Autodesk Inventor part; units mm, degrees
ref_plane "YZ Plane" through (0, 0, 0) normal (1, 0, 0) x (0, 1, 0)
ref_plane "XZ Plane" through (0, 0, 0) normal (0, 1, 0) x (-1, 0, 0)
ref_plane "XY Plane" through (0, 0, 0) normal (0, 0, 1) x (1, 0, 0)
sketch "Sketch1" plane through (0, 0, 0) normal (0, 0, 1) x (1, 0, 0)
  line L0 (0, 0) -> (60, 0)
  line L1 (60, 0) -> (60, 60)
  line L2 (60, 60) -> (0, 60)
  line L3 (0, 60) -> (0, 0)
  dimension "d0" = 60
  dimension "d1" = 60
extrude "Extrusion1" add sketch "Sketch1" along normal blind 22
sketch "Sketch2" plane through (0, 0, 0) normal (0, 0, -1) x (-1, 0, 0)
  line L0 (0, 10.6066) -> (-10.6066, 0)
  line L1 (0, 10.6066) -> (0, 0)
  line L2 (0, 0) -> (-10.6066, 0)
  line L3 (0, 60) -> (-10.6066, 60)
  line L4 (-10.6066, 60) -> (0, 49.3934)
  line L5 (0, 49.3934) -> (0, 60)
  line L6 (-49.3934, 60) -> (-60, 60)
  line L7 (-60, 60) -> (-60, 49.3934)
  line L8 (-49.3934, 60) -> (-60, 49.3934)
  line L9 (-49.3934, 0) -> (-60, 0)
  line L10 (-60, 0) -> (-60, 10.6066)
  line L11 (-49.3934, 0) -> (-60, 10.6066)
  dimension "d4" = 15
  dimension "d7" = 15
  dimension "d8" = 15
  dimension "d9" = 15
extrude "Extrusion2" cut sketch "Sketch2" against normal blind 13
sketch "Sketch7" plane through (0, 0, 22) normal (0, 0, 1) x (1, 0, 0)
  circle A0 centre (45.5887, 39) radius 8 construction
  circle A1 centre (14.4113, 39) radius 8 construction
  line L0 (22, 49.3156) -> (26.1411, 33.8608) construction
  line L1 (26.1411, 33.8608) -> (16.4818, 31.2726)
  line L2 (12.3407, 46.7274) -> (22, 49.3156)
  line L3 (33.8589, 33.8608) -> (38, 49.3156) construction
  line L4 (38, 49.3156) -> (47.6593, 46.7274)
  line L5 (33.8589, 33.8608) -> (43.5182, 31.2726)
  line L6 (22, 49.3156) -> (38, 49.3156) construction
  line L7 (26.1411, 33.8608) -> (33.8589, 33.8608)
  arc A2 (12.3407, 46.7274) -> (16.4818, 31.2726) centre (14.4113, 39) ccw
  arc A3 (43.5182, 31.2726) -> (47.6593, 46.7274) centre (45.5887, 39) ccw
  line L8 (60, 60) -> (0, 60)
  arc A4 (38, 49.3156) -> (22, 49.3156) centre (30, 19.4592) ccw
  point P0 (0, 0)
  point P1 (30, 49.3156)
  point P2 (30, 60)
  dimension "d28" = 16
  dimension "d29" = 16
  dimension "d30" = 16
  dimension "d31" = 10
  dimension "d32" = 10
  dimension "d33" = 16
  dimension "d34" = 16
  dimension "d36" = 75
  dimension "d37" = 21
extrude "Extrusion7" add sketch "Sketch7" along normal blind 34
sketch "Sketch8" plane through (10.6066, 0, 13) normal (-0.7071, -0.7071, 0) x (-0.7071, 0.7071, 0)
  circle A0 centre (7.5, 9) radius 1.5
  line L0 (0, 13) -> (15, 13)
  point P0 (7.5, 13)
  point P1 (7.5, 13)
  dimension "d40" = 3
  dimension "d41" = 4
extrude "Extrusion8" cut sketch "Sketch8" against normal through all
sketch "Sketch9" plane through (60, 10.6066, 13) normal (0.7071, -0.7071, 0) x (-0.7071, -0.7071, 0)
  circle A0 centre (7.5, 9) radius 1.5
  line L0 (0, 13) -> (15, 13)
  point P0 (49.9264, 13)
  point P1 (7.5, 13)
  dimension "d44" = 3
  dimension "d45" = 4
extrude "Extrusion9" cut sketch "Sketch9" against normal through all
sketch "Sketch10" plane through (0, 0, 56) normal (0, 0, 1) x (1, 0, 0)
  line L0 (22, 49.3156) -> (12.3407, 46.7274) construction
  arc A0 (12.3407, 46.7274) -> (16.4818, 31.2726) centre (14.4113, 39) ccw construction
  line L1 (16.4818, 31.2726) -> (26.1411, 33.8608) construction
  line L2 (26.1411, 33.8608) -> (33.8589, 33.8608) construction
  line L3 (33.8589, 33.8608) -> (43.5182, 31.2726) construction
  arc A1 (43.5182, 31.2726) -> (47.6593, 46.7274) centre (45.5887, 39) ccw construction
  line L4 (47.6593, 46.7274) -> (38, 49.3156) construction
  arc A2 (38, 49.3156) -> (22, 49.3156) centre (30, 19.4592) ccw construction
  circle A3 centre (14.4113, 39) radius 1.75
  circle A4 centre (45.5887, 39) radius 1.75
  circle A5 centre (30, 46.8608) radius 1.75
  point P0 (0, 0)
  point P1 (30, 33.8608)
  dimension "d48" = 3.5
  dimension "d49" = 3.5
  dimension "d50" = 3.5
  dimension "d51" = 13
extrude "Extrusion10" cut sketch "Sketch10" against normal blind 29
properties part number "Base" material "ABS Plastic"
CAD build for the part. Positions are in the model's coordinates, mm. A direction names the side the tool comes from. Give positions to 0.01 mm unless a question says otherwise; leave off trailing zeros. Write each loop counter-clockwise with the first axis right and the second up, starting at its lowest first coordinate (ties: lowest second). Pieces come first, ordered by that corner, then holes. Notation, with made-up numbers: M -25,27.5 L 19,27.5 A31 cw 19,60.5 Z; hole C 2.25,82.25 d11. An arc over 180 degrees is marked long. Return JSON: item names as keys, results as strings. Group by question number.
(1) Mould opens along X. For faces 1 (the face through (3, 3, 13)), 2 (the face through (17.254, 41.605, 2.735)), 3 (the face through (42.76, 48.04, 38.76)), 4 (the face through (14, 37.3, 41.7)) say: pulls with the +X half, pulls with the -X half, needs draft (parallel to the pull), parting line crosses it, or undercut.
(2) Band-saw the part on A-A (z = 33.5). Give the cut face in (x, y).
(3) Band-saw the part on B-B (y = 39). State how many separate pieces and enclosed holes the cut face has, and give its area (3 significant figures).
(4) 3-axis set-ups, long thin cutter, end or side, ignore diameter. For faces 5 (the face through (46, 39, 27)), 6 (the face through (57, 3, 13)), 7 (the face through (29.89, 50.37, 38.76)), 8 (the face through (56, 56, 13)): which of +Z, -Z, +X, -X, +Y, -Y reach the whole face in a straight line?
(5) Flat gauge pins, fed straight in: pin 1 Ø4 at (x, z) = (39.5, 43) entering from +Y; pin 2 Ø1.5 at (x, z) = (41, 34.5) entering from +Y; pin 3 Ø1.5 at (x, z) = (34.5, 42.5) entering from -Y. Where does each tip first touch, or does it go through?
(6) Drill centre lines: L1, parallel to Y at x = 30, z = 50; L2, parallel to Z at x = 54, y = 6; L3, parallel to Z at x = 37, y = 30.5. Where is each one in solid material? Low to high. Write a range as [from, to].
Entries:
{
 "1": {"face 1": "needs draft", "face 2": "undercut", "face 3": "pulls with the +X half", "face 4": "undercut"},
 "2": {"outline": "M 12.34,46.73 A8 ccw 16.48,31.27 L 26.14,33.86 L 33.86,33.86 L 43.52,31.27 A8 ccw 47.66,46.73 L 38,49.32 A30.91 ccw 22,49.32 Z; hole C 14.41,39 d3.5; hole C 30,46.86 d3.5; hole C 45.59,39 d3.5"},
 "3": {"separate pieces": "1", "enclosed holes": "2", "area": "2,700 mm^2"},
 "4": {"face 5": "+Z", "face 6": "-Z, +X, -Y", "face 7": "+Z, +Y", "face 8": "-Z, +X, +Y"},
 "5": {"pin 1": "stops at y = 49.45", "pin 2": "stops at y = 48.71", "pin 3": "stops at y = 33.49"},
 "6": {"L1": "y = [33.86, 45.11], [48.61, 50.37]", "L2": "z = [0, 2.5], [5.5, 22]", "L3": "z = [0, 22]"}
}
